The listing builds one solid part. Answer for the finished solid, in the listing's coordinates (mm). A direction names the side the tool comes from. Coordinates: 2 decimals unless noted, no trailing zeros. Order: outer loops, then holes, each group sorted by start corner. A loop starts at its lowest first (then second) coordinate and runs counter-clockwise, first axis right, second up. Notation, with made-up numbers: (-32.75, -23.75) -> (10.25, -23.75) arc R17 ccw to (10.25, 1.25) -> close; hole circle Ø1 at (87.5, 13.25). An arc over 180 degrees is marked (long way). Answer in a Markdown table with one row per item.
```python
from build123d import *

# Parameters (mm, degrees)
SKETCH1_W           = 25.4
SKETCH1_H           = 25.4
SKETCH1_W_2         = 19.05
SKETCH1_H_2         = 19.05
BOSS_EXTRUDE1_DEPTH = 63.5
SKETCH2_R           = 2.0193
CUT_EXTRUDE1_DEPTH  = 63.5
SKETCH3_R           = 2.0193
CUT_EXTRUDE2_DEPTH  = 63.5
CUT_EXTRUDE3_DEPTH  = 28.702
SKETCH5_W           = 25.4
SKETCH5_H           = 25.4
CUT_EXTRUDE4_DEPTH  = 12.7


with BuildPart() as part:
    # Sketch1 → Boss-Extrude1 (new body)
    with BuildSketch(Plane.XY):
        with Locations((12.7, 12.7)):
            Rectangle(SKETCH1_W, SKETCH1_H)
        with Locations((12.7, 12.7)):
            Rectangle(SKETCH1_W_2, SKETCH1_H_2, mode=Mode.SUBTRACT)
    extrude(amount=BOSS_EXTRUDE1_DEPTH)

    # Sketch2 → Cut-Extrude1 (cut)
    with BuildSketch(Plane(origin=(0, 25.4, 0), x_dir=(1, 0, 0), z_dir=(0, 1, 0))):
        with Locations((12.7, -50.8)):
            Circle(SKETCH2_R)
        with Locations((12.7, -38.1)):
            Circle(SKETCH2_R)
        with Locations((12.7, -25.4)):
            Circle(SKETCH2_R)
        with Locations((12.7, -12.7)):
            Circle(SKETCH2_R)
    extrude(amount=-CUT_EXTRUDE1_DEPTH, mode=Mode.SUBTRACT)

    # Sketch3 → Cut-Extrude2 (cut)
    with BuildSketch(Plane(origin=(25.4, 0, 0), x_dir=(0, 0, -1), z_dir=(1, 0, 0))):
        with Locations((-50.8, 12.7)):
            Circle(SKETCH3_R)
        with Locations((-38.1, 12.7)):
            Circle(SKETCH3_R)
        with Locations((-25.4, 12.7)):
            Circle(SKETCH3_R)
        with Locations((-12.7, 12.7)):
            Circle(SKETCH3_R)
    extrude(amount=-CUT_EXTRUDE2_DEPTH, mode=Mode.SUBTRACT)

    # Sketch4 → Cut-Extrude3 (cut)
    with BuildSketch(Plane(origin=(25.4, 0, 0), x_dir=(0, 0, -1), z_dir=(1, 0, 0))):
        Polygon((-9.033825791, 19.05), (-16.366174209, 19.05), (-20.032348419, 12.7), (-16.366174209, 6.35), (-9.033825791, 6.35), (-5.367651581, 12.7), align=None)
    extrude(amount=-CUT_EXTRUDE3_DEPTH, mode=Mode.SUBTRACT)

    # Sketch5 → Cut-Extrude4 (cut)
    with BuildSketch(Plane.XY.offset(63.5)):
        with Locations((12.7, 12.7)):
            Rectangle(SKETCH5_W, SKETCH5_H)
    extrude(amount=-CUT_EXTRUDE4_DEPTH, mode=Mode.SUBTRACT)


solid = part.part
```
(1) A cutting plane is placed at A-A, the plane y = 21.25. Determine the outline of the cut face in (x, z) (3 decimals).
Check values:
| item | result |
|---|---|
| outline | (0, 0) -> (3.175, 0) -> (3.175, 50.8) -> (0, 50.8) -> close; (22.225, 0) -> (25.4, 0) -> (25.4, 50.8) -> (22.225, 50.8) -> close |
(2) Find the intervals of material crossed by line 1 along Z through (x, y) = (12.7, 1.9); line 2 along X through (y, z) = (10, 29.5) (3 decimals), in increasing order. Write a range as from..to.
Check values:
| item | result |
|---|---|
| line 1 | 0..10.68, 14.72..23.38, 27.42..36.08, 40.12..48.78 |
| line 2 | 0..3.175, 22.225..25.4 |
(3) Flat-ended cylindrical pins translate along their axes: pin 1 (12 mm diameter, centred on x = 8.5, z = 41.5, fed in from -Y); pin 2 (10 mm diameter, centred on x = 10, y = 15.5, fed in from +Z). Find the tip coordinate at first contact, or state that the pin passes through.
Check values:
| item | result |
|---|---|
| pin 1 | y = 0 |
| pin 2 | through |
(4) For a pull along Z with two mould halves and no side action, classify faces 3 (the flat face through (21, 23, 50.8)), 4 (the flat face through (2, 19.05, 13)), 5 (the flat face through (22.225, 10, 25)), 6 (the flat face through (23.835, 15.831, 7.175)) as released by +Z, released by -Z, zero draft, split by the parting line, or undercut.
Check values:
| item | result |
|---|---|
| face 3 | released by +Z |
| face 4 | undercut |
| face 5 | zero draft |
| face 6 | undercut |
(5) A cutting plane is placed at C-C, the plane x = 12.7. Count the separate pieces of the cut face and the enclosed holes in it, then the cut area to 3 significant figures.
Check values:
| item | result |
|---|---|
| separate pieces | 8 |
| enclosed holes | 0 |
| area | 233 mm² |
(6) Which of the six approach directions +Z, -Z, +X, -X, +Y, -Y give full straight-line access (tool end or side, diameter ignored) to faces 1 (the flat face through (23.835, 15.919, 18.174)), 2 (the flat face through (21, 3, 50.8))?
Check values:
| item | result |
|---|---|
| face 1 | +X, -X |
| face 2 | +Z, +X, -X, +Y, -Y |
(7) A cutting plane is placed at B-B, the plane z = 25.4. Determine the outline of the cut face in (x, y) (3 decimals), then the cut area to 3 significant figures.
Check values:
| item | result |
|---|---|
| outline | (0, 0) -> (10.681, 0) -> (10.681, 3.175) -> (3.175, 3.175) -> (3.175, 10.681) -> (0, 10.681) -> close; (0, 14.719) -> (3.175, 14.719) -> (3.175, 22.225) -> (10.681, 22.225) -> (10.681, 25.4) -> (0, 25.4) -> close; (14.719, 0) -> (25.4, 0) -> (25.4, 10.681) -> (22.225, 10.681) -> (22.225, 3.175) -> (14.719, 3.175) -> close; (14.719, 22.225) -> (22.225, 22.225) -> (22.225, 14.719) -> (25.4, 14.719) -> (25.4, 25.4) -> (14.719, 25.4) -> close |
| area | 231 mm² |
